from build123d import *

# Parameters (mm, degrees)
SKETCH_2_W      = 80.819107854
SKETCH_2_H      = 57.34
SKETCH_2_R      = 1.6
EXTRUDE_1_DEPTH = 1.5
FILLET_1_R      = 2


with BuildPart() as part:
    # 스케치2 → 보스-돌출1 (new body)
    with BuildSketch(Plane(origin=(0, 0, 0), x_dir=(1, 0, 0), z_dir=(0, 1, 0))):
        with Locations((-2.909553927, 0)):
            Rectangle(SKETCH_2_W, SKETCH_2_H)
        with Locations(Location((-37.73627176, 24.13, 0), (0, 0, 270))):
            Circle(SKETCH_2_R, mode=Mode.SUBTRACT)
        with Locations(Location((-37.73627176, -24.13, 0), (0, 0, 90))):
            Circle(SKETCH_2_R, mode=Mode.SUBTRACT)
        with BuildLine():
            ThreePointArc((31.36, 8.89), (32.96, 7.29), (34.56, 8.89))
            ThreePointArc((34.56, 8.89), (32.96, 10.49), (31.36, 8.89))
        make_face(mode=Mode.SUBTRACT)
        with BuildLine():
            ThreePointArc((31.36, -19.05), (32.96, -20.65), (34.56, -19.05))
            ThreePointArc((34.56, -19.05), (32.96, -17.45), (31.36, -19.05))
        make_face(mode=Mode.SUBTRACT)
        with BuildLine():
            ThreePointArc((-20.71, -24.13), (-19.11, -25.73), (-17.51, -24.13))
            ThreePointArc((-17.51, -24.13), (-19.11, -22.53), (-20.71, -24.13))
        make_face(mode=Mode.SUBTRACT)
        with BuildLine():
            ThreePointArc((-20.71, 24.13), (-19.11, 25.73), (-17.51, 24.13))
            ThreePointArc((-17.51, 24.13), (-19.11, 22.53), (-20.71, 24.13))
        make_face(mode=Mode.SUBTRACT)
    extrude(amount=EXTRUDE_1_DEPTH)

    # 필렛1
    fillet_1_edges = [part.edges().sort_by_distance(p)[0] for p in [
        (37.5, 0.75, 28.67),
        (-43.319107854, 0.75, 28.67),
        (-43.319107854, 0.75, -28.67),
        (37.5, 0.75, -28.67),
    ]]
    fillet(fillet_1_edges, radius=FILLET_1_R)


solid = part.part
Can you work these out from the model? Positions are in its coordinate system, mm. Round coordinates to 2 decimals unless told otherwise and drop trailing zeros. Order: outer loops, then holes, each group sorted by start corner. A loop starts at its lowest first (then second) coordinate and runs counter-clockwise, first axis right, second up. Notation, with made-up numbers: M -30.5,13.25 L 10.5,13.25 A10 cw 10.5,21.25 Z; hole C 34.25,21 d2. An arc over 180 degrees is marked long. Use a Markdown table: item, result.
1) If I drill on line 1 along Z through (x, y) = (32.96, 0.3); line 2 along X through (y, z) = (1, 24.13); line 3 along Z through (x, y) = (-19.11, 0.8), over which ranges is the centre line in solid material (lowest first)?
Geometry says:
| item | result |
|---|---|
| line 1 | z = -28.67 to -10.49, -7.29 to 17.45, 20.65 to 28.67 |
| line 2 | x = -43.32 to -39.34, -36.14 to -20.71, -17.51 to 37.5 |
| line 3 | z = -28.67 to -25.73, -22.53 to 22.53, 25.73 to 28.67 |
2) I'm going to push a flat-ended pin straight in: P1, Ø1.5, axis at x = -9, z = 7, coming from the -Y side. Where does the tip first touch, or does it pass through?
Geometry says:
| item | result |
|---|---|
| P1 | stops at y = 0 |
3) Imagine slicing it at A-A (z = 19.05). List the corners of the cut face in (x, y) for me, then the cut area to 3 significant figures.
Geometry says:
| item | result |
|---|---|
| outline | M -43.32,0 L 31.36,0 L 31.36,1.5 L -43.32,1.5 Z; M 34.56,0 L 37.5,0 L 37.5,1.5 L 34.56,1.5 Z |
| area | 116 mm² |
4) Imagine slicing it at C-C (z = -24.13). List the corners of the cut face in (x, y) for me, then the cut area to 3 significant figures.
Geometry says:
| item | result |
|---|---|
| outline | M -43.32,0 L -39.34,0 L -39.34,1.5 L -43.32,1.5 Z; M -36.14,0 L -20.71,0 L -20.71,1.5 L -36.14,1.5 Z; M -17.51,0 L 37.5,0 L 37.5,1.5 L -17.51,1.5 Z |
| area | 112 mm² |
5) If we mould it in two halves opening along X, with no side actions, what happens to faces 1 (the face through (36.9, 0.8, -28.1)), 2 (the face through (-42.75, 0.76, -28.07)), 3 (the face through (-17.6, 0.7, 23.6))? For each: +X half, -X half, draft (parallel to the pull), parting line (faces both ways), or undercut.
Geometry says:
| item | result |
|---|---|
| face 1 | +X half |
| face 2 | -X half |
| face 3 | undercut |
6) Imagine slicing it at B-B (x = -19.11). List the corners of the cut face in (y, z) for me, then the cut area to 3 significant figures.
Geometry says:
| item | result |
|---|---|
| outline | M 0,-28.67 L 1.5,-28.67 L 1.5,-25.73 L 0,-25.73 Z; M 0,-22.53 L 1.5,-22.53 L 1.5,22.53 L 0,22.53 Z; M 0,25.73 L 1.5,25.73 L 1.5,28.67 L 0,28.67 Z |
| area | 76.4 mm² |
